from build123d import *

# Parameters (mm, degrees)
BOSS_EXTRUDE1_DEPTH = 4.6
CUT_EXTRUDE1_DEPTH  = 5.6


with BuildPart() as part:
    # Sketch1 → Boss-Extrude1 (new body)
    with BuildSketch(Plane.XY):
        Polygon((47.4, 11.783577493), (52, 11.783577493), (52, -11.783577493), (47.4, -11.783577493), (47.4, -47.7), (11.483577493, -47.7), (11.483577493, -52.3), (-12.083577493, -52.3), (-12.083577493, -47.7), (-48, -47.7), (-48, -11.783577493), (-52.6, -11.783577493), (-52.6, 11.783577493), (-48, 11.783577493), (-48, 47.7), (-12.083577493, 47.7), (-12.083577493, 52.3), (11.483577493, 52.3), (11.483577493, 47.7), (47.4, 47.7), align=None)
    extrude(amount=BOSS_EXTRUDE1_DEPTH)

    # Sketch2 → Cut-Extrude1 (cut, through all)
    with BuildSketch(Plane(origin=(0, 0, 0), x_dir=(-1, 0, 0), z_dir=(0, 0, -1))):
        Polygon((9.417835971, -37.7), (9.417835971, -33.1), (-6.62560911, -33.1), (-6.62560911, -37.7), (-37.7, -37.7), (-37.7, -9.417835971), (-33.1, -9.417835971), (-33.1, 6.62560911), (-37.7, 6.62560911), (-37.7, 37.7), (-9.417835971, 37.7), (-9.417835971, 33.1), (6.62560911, 33.1), (6.62560911, 37.7), (37.7, 37.7), (37.7, 9.417835971), (33.1, 9.417835971), (33.1, -6.62560911), (37.7, -6.62560911), (37.7, -37.7), align=None)
    extrude(amount=-CUT_EXTRUDE1_DEPTH, mode=Mode.SUBTRACT)


solid = part.part
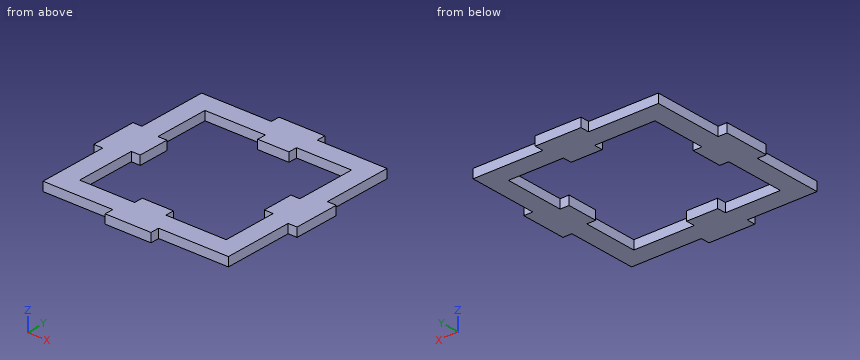
The model under review builds one solid part; all positions refer to its coordinate system, in mm. Coordinates: 2 decimals unless noted, no trailing zeros. Write each loop counter-clockwise with the first axis right and the second up, starting at its lowest first coordinate (ties: lowest second). Pieces come first, ordered by that corner, then holes. Notation, with made-up numbers: M 1,61.25 L 44,61.25 A12 cw 44,65.25 Z; hole C 75.5,-39 d4. An arc over 180 degrees is marked long. Put each result on its own line as item: value.
1) Clearance check with flat-ended pins moving along their axes: pin 1 Ø1 at (x, z) = (13.5, 4) entering from -Y; pin 2 Ø2.5 at (x, z) = (-50.5, 2.5) entering from +Y; pin 3 Ø1.4 at (x, z) = (-50, 2) entering from -Y. State where each tip first meets the part, or that it passes through.
Computed:
pin 1: stops at y = -47.7
pin 2: stops at y = 11.78
pin 3: stops at y = -11.78
2) Add section A-A on y = -17.5. Give the boundary of the cut face in (x, z), then the cut area to 3 significant figures.
Computed:
outline: M -48,0 L -37.7,0 L -37.7,4.6 L -48,4.6 Z; M 37.7,0 L 47.4,0 L 47.4,4.6 L 37.7,4.6 Z
area: 92.0 mm2
3) Add section B-B on x = 15. Give the boundary of the cut face in (y, z), then the cut area to 3 significant figures.
Computed:
outline: M -47.7,0 L -37.7,0 L -37.7,4.6 L -47.7,4.6 Z; M 37.7,0 L 47.7,0 L 47.7,4.6 L 37.7,4.6 Z
area: 92.0 mm2
4) Wall thickness on probe 1 along Y at (x, z) = (-37, 3.75); probe 2 along Y at (x, z) = (36.5, 0.3); probe 3 along X at (y, z) = (-12, 2.3): over which ranges is each line inside the solid? List them lowest first. Write a range as [from, to].
Computed:
probe 1: y = [-47.7, -37.7], [-6.63, 9.42], [37.7, 47.7]
probe 2: y = [-47.7, -37.7], [-9.42, 6.63], [37.7, 47.7]
probe 3: x = [-48, -37.7], [37.7, 47.4]
5) Add section C-C on y = 36.5. Give the boundary of the cut face in (x, z).
Computed:
outline: M -48,0 L -37.7,0 L -37.7,4.6 L -48,4.6 Z; M -6.63,0 L 9.42,0 L 9.42,4.6 L -6.63,4.6 Z; M 37.7,0 L 47.4,0 L 47.4,4.6 L 37.7,4.6 Z
